Geometry check sheet. Reference: the model listing, model coordinates, mm. Face numbers are marked on the shaded views. A direction names the side the tool comes from. Give positions to 0.01 mm unless a question says otherwise; leave off trailing zeros. Loops run counter-clockwise (first coordinate to the right, second up) from the corner with the lowest first, then second, coordinate; pieces in that order, holes last. Notation, with made-up numbers: (88, 19) - (115, 19) arc R15 ccw to (115, 36) - close; hole circle Ø7 at (10, 23.25). An arc over 180 degrees is marked (long way). Use a Markdown table: item, result. Add a question column.
1. Cross-section at B-B on z = 5. Enter the section's corners in (x, y) (3 decimals).
2. Cross-section at D-D on x = -20.5. Enter the section's corners in (y, z) (3 decimals).
3. Material ranges on L1, parallel to Z at x = -20.5, y = 17.2 (3 decimals); L2, parallel to X at y = 12.5, z = -10 (3 decimals); L3, parallel to Z at x = -20.5, y = 18.75, recorded low to high.
4. Cross-section at C-C on z = -11. Enter the section's corners in (x, y) (3 decimals).
5. Draft check along X on the marked faces 1, 2, 3 and 4. Enter one of: pulls with the +X half, pulls with the -X half, needs draft (parallel to the pull), parting line crosses it, or undercut.
6. Cross-section at A-A on x = 5.5. Enter the section's corners in (y, z) (3 decimals), and give its area (3 significant figures).
7. Set-up check for the marked faces 5 and 6: record each of +Z, -Z, +X, -X, +Y, -Y from which the full face is reachable in a straight line by a thin tool's end or side.
8. Depth check by flat-ended pin: P1, Ø1, axis at x = 28, z = -21.5, coming from the -Y side; P2, Ø2.5, axis at x = 9, y = 19.5, coming from the -Z side; P3, Ø3, axis at x = -8, y = 8.5, coming from the +Z side. Enter the tip coordinate at first touch or a pass-through.
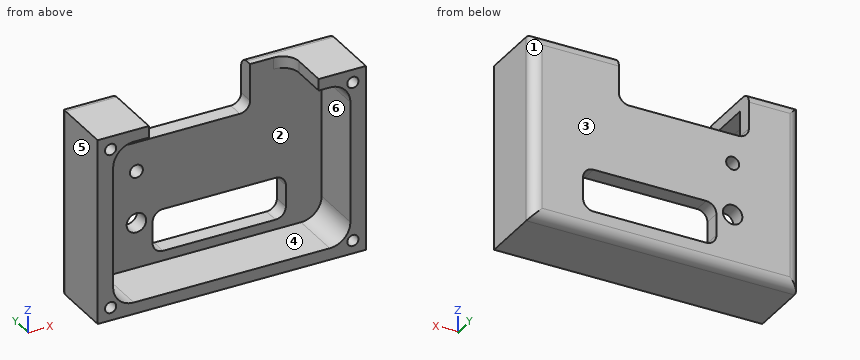
from build123d import *

# Parameters (mm, degrees)
SKETCH1_W                 = 82.55
SKETCH1_H                 = 57.15
BOSS_EXTRUDE1_DEPTH       = 21.018
CUT_EXTRUDE1_DEPTH        = 16
F_8_32_TAPPED_HOLE1_D     = 3.4544
F_8_32_TAPPED_HOLE1_DEPTH = 10.708
F_8_32_TAPPED_HOLE1_TIP   = 1.037806461
FILLET1_R                 = 3.175
SKETCH6_R                 = 3
SKETCH6_R_2               = 2
CUT_EXTRUDE2_DEPTH        = 22.018
CUT_EXTRUDE3_REACH        = 59.15


with BuildPart() as part:
    # Sketch1 → Boss-Extrude1 (new body)
    with BuildSketch(Plane(origin=(0, 0, 0), x_dir=(1, 0, 0), z_dir=(0, 1, 0))):
        Rectangle(SKETCH1_W, SKETCH1_H)
    extrude(amount=BOSS_EXTRUDE1_DEPTH)

    # Sketch2 → Cut-Extrude1 (cut)
    with BuildSketch(Plane(origin=(0, 0, 0), x_dir=(1, 0, 0), z_dir=(0, 1, 0))):
        with BuildLine():
            Line((30.15, -25), (-30.15, -25))
            ThreePointArc((-30.15, -25), (-34.640128061, -23.140128061), (-36.5, -18.65))
            Line((-36.5, -18.65), (-36.5, 18.65))
            ThreePointArc((-36.5, 18.65), (-34.640128061, 23.140128061), (-30.15, 25))
            Line((-30.15, 25), (30.15, 25))
            ThreePointArc((30.15, 25), (34.640128061, 23.140128061), (36.5, 18.65))
            Line((36.5, 18.65), (36.5, -18.65))
            ThreePointArc((36.5, -18.65), (34.640128061, -23.140128061), (30.15, -25))
        make_face()
    extrude(amount=CUT_EXTRUDE1_DEPTH, mode=Mode.SUBTRACT)

    # #8-32 Tapped Hole1
    with Locations(Plane(origin=(0, 0, 0), x_dir=(-1, 0, 0), z_dir=(0, -1, 0))):
        with Locations((37.275, -24.575), (37.275, 24.575), (-37.275, -24.575), (-37.275, 24.575)):
            Hole(F_8_32_TAPPED_HOLE1_D / 2, depth=F_8_32_TAPPED_HOLE1_DEPTH)
            with Locations((0, 0, -(F_8_32_TAPPED_HOLE1_DEPTH + F_8_32_TAPPED_HOLE1_TIP / 2))):  # 118° drill point
                Cone(0, F_8_32_TAPPED_HOLE1_D / 2, F_8_32_TAPPED_HOLE1_TIP, mode=Mode.SUBTRACT)

    # Fillet1
    fillet1_edges = [part.edges().sort_by_distance(p)[0] for p in [
        (41.275, 21.018, 0),
        (0, 21.018, -28.575),
        (-41.275, 21.018, 0),
        (0, 21.018, 28.575),
    ]]
    fillet(fillet1_edges, radius=FILLET1_R)

    # Sketch6 → Cut-Extrude2 (cut, through all)
    with BuildSketch(Plane(origin=(0, 21.018, 0), x_dir=(1, 0, 0), z_dir=(0, 1, 0))):
        with Locations((-20.5, 11)):
            Circle(SKETCH6_R)
        with Locations((-20.5, -5)):
            Circle(SKETCH6_R_2)
        with BuildLine():
            Line((-12.325, 9), (22.325, 9))
            ThreePointArc((22.325, 9), (24.57006403, 9.92993597), (25.5, 12.175))
            Line((25.5, 12.175), (25.5, 18.825))
            ThreePointArc((25.5, 18.825), (24.57006403, 21.07006403), (22.325, 22))
            Line((22.325, 22), (-12.325, 22))
            ThreePointArc((-12.325, 22), (-14.57006403, 21.07006403), (-15.5, 18.825))
            Line((-15.5, 18.825), (-15.5, 12.175))
            ThreePointArc((-15.5, 12.175), (-14.57006403, 9.92993597), (-12.325, 9))
        make_face()
        with BuildLine():
            Line((-25.5, -28.575), (14.5, -28.575))
            Line((14.5, -28.575), (14.5, -17.175))
            ThreePointArc((14.5, -17.175), (13.57006403, -14.92993597), (11.325, -14))
            Line((11.325, -14), (-22.325, -14))
            ThreePointArc((-22.325, -14), (-24.57006403, -14.92993597), (-25.5, -17.175))
            Line((-25.5, -17.175), (-25.5, -28.575))
        make_face()
    extrude(amount=-CUT_EXTRUDE2_DEPTH, mode=Mode.SUBTRACT)

    # Sketch7 → Cut-Extrude3 (cut, up to next)
    with BuildSketch(Plane.XY.offset(28.575), mode=Mode.PRIVATE) as cut_extrude3_sk1:
        with BuildLine():
            Line((21.75, 16), (14.5, 16))
            Line((14.5, 16), (14.5, 0))
            Line((14.5, 0), (26.75, 0))
            Line((26.75, 0), (26.75, 11))
            ThreePointArc((26.75, 11), (25.285533906, 14.535533906), (21.75, 16))
        make_face()
    cut_extrude3_tool1 = extrude(cut_extrude3_sk1.sketch, amount=-CUT_EXTRUDE3_REACH, mode=Mode.PRIVATE) & part.part
    add(cut_extrude3_tool1.solids().sort_by_distance((20.484055, 7.806287, 28.575))[0], mode=Mode.SUBTRACT)


solid = part.part
Values found:
| question | item | result |
|---|---|---|
| 1 | outline | (-41.275, 0) - (-36.5, 0) - (-36.5, 16) - (-22.5, 16) - (-22.5, 21.018) - (-38.1, 21.018) arc R3.175 ccw to (-41.275, 17.843) - close; (-18.5, 16) - (36.5, 16) - (36.5, 0) - (41.275, 0) - (41.275, 17.843) arc R3.175 ccw to (38.1, 21.018) - (-18.5, 21.018) - close |
| 2 | outline | (0, -28.575) - (17.843, -28.575) arc R3.175 ccw to (21.018, -25.4) - (21.018, -14) - (16, -14) - (16, -25) - (0, -25) - close; (16, -8) - (21.018, -8) - (21.018, 3) - (16, 3) - close; (16, 7) - (21.018, 7) - (21.018, 14) - (16, 14) - close |
| 3 | L1 | z = -28.575 to -14, -8 to 3, 7 to 14 |
| 3 | L2 | x = -41.275 to -36.5, 36.5 to 41.275 |
| 3 | L3 | z = -28.44 to -14, -8 to 3, 7 to 14 |
| 4 | outline | (-41.275, 0) - (-36.5, 0) - (-36.5, 16) - (-23.5, 16) - (-23.5, 21.018) - (-38.1, 21.018) arc R3.175 ccw to (-41.275, 17.843) - close; (-17.5, 16) - (-15.275, 16) - (-15.275, 21.018) - (-17.5, 21.018) - close; (25.275, 16) - (36.5, 16) - (36.5, 0) - (41.275, 0) - (41.275, 17.843) arc R3.175 ccw to (38.1, 21.018) - (25.275, 21.018) - close |
| 5 | face 1 | pulls with the +X half |
| 5 | face 2 | undercut |
| 5 | face 3 | needs draft |
| 5 | face 4 | undercut |
| 6 | outline | (0, -28.575) - (17.843, -28.575) arc R3.175 ccw to (21.018, -25.4) - (21.018, -22) - (16, -22) - (16, -25) - (0, -25) - close; (16, -9) - (21.018, -9) - (21.018, 14) - (16, 14) - close |
| 6 | area | 203 mm2 |
| 7 | face 5 | +Z, -Z, -X, +Y, -Y |
| 7 | face 6 | -Y |
| 8 | P1 | stops at y = 16 |
| 8 | P2 | stops at z = -28.55 |
| 8 | P3 | stops at z = -25 |
